```python
from build123d import *

# Parameters (mm, degrees)
BOSS_EXTRUDE1_DEPTH = 400
BOSS_EXTRUDE2_DEPTH = 10
SKETCH3_R           = 43.000999871
CUT_EXTRUDE1_DEPTH  = 447.360216168
BOSS_EXTRUDE3_DEPTH = 7
SKETCH5_R           = 1.75
CUT_EXTRUDE2_DEPTH  = 33
SKETCH6_W           = 36.000000185
SKETCH6_H           = 60
BOSS_EXTRUDE4_DEPTH = 5
SKETCH7_W           = 7.24997928
SKETCH7_H           = 16
BOSS_EXTRUDE5_DEPTH = 53
SKETCH8_W           = 12.24997928
SKETCH8_H           = 60
BOSS_EXTRUDE6_DEPTH = 5
FILLET1_R           = 5
SKETCH10_W          = 20.000000185
SKETCH10_H          = 40
BOSS_EXTRUDE7_DEPTH = 7.24997928
CUT_EXTRUDE3_DEPTH  = 6
CUT_EXTRUDE4_DEPTH  = 68.845857758
SKETCH12_R          = 4.5
CUT_EXTRUDE5_DEPTH  = 16
CHAMFER2_SIZE       = 5
CHAMFER3_SIZE       = 5
SKETCH13_R          = 6.5
SKETCH13_R_2        = 4.5
BOSS_EXTRUDE8_DEPTH = 2
FILLET2_R           = 1


with BuildPart() as part:
    # Sketch1 → Boss-Extrude1 (new body)
    with BuildSketch(Plane(origin=(0, 200, 0), x_dir=(1, 0, 0), z_dir=(0, 1, 0))):
        with BuildLine():
            Line((1e-09, -3.855700002), (0.25, -4.00003757))
            Line((0.25, -4.00003757), (9.078700232, -4.00003757))
            ThreePointArc((9.078700232, -4.00003757), (9.652725366, -4.114218268), (10.139360377, -4.439377387))
            Line((10.139360377, -4.439377387), (12.500020747, -6.800037757))
            Line((12.500020747, -6.800037757), (12.500020747, -9.500037757))
            Line((12.500020747, -9.500037757), (13.00002072, -10.000037755))
            Line((13.00002072, -10.000037755), (17.00002072, -10.000037755))
            Line((17.00002072, -10.000037755), (17.500020747, -9.500037752))
            Line((17.500020747, -9.500037752), (17.500020747, -5.500037752))
            Line((17.500020747, -5.500037752), (17.00002075, -5.0000377))
            Line((17.00002075, -5.0000377), (14.30002072, -5.0000377))
            Line((14.30002072, -5.0000377), (14.085807141, -4.785824121))
            ThreePointArc((14.085807141, -4.785824121), (13.652261651, -4.136977442), (13.50002072, -3.371610598))
            Line((13.50002072, -3.371610598), (13.50002072, -0.30003757))
            Line((13.50002072, -0.30003757), (13.20002072, -3.757e-05))
            Line((13.20002072, -3.757e-05), (7.50002072, -3.757e-05))
            Line((7.50002072, -3.757e-05), (7.40002072, -0.10003757))
            Line((7.40002072, -0.10003757), (-7.40002072, -0.10003757))
            Line((-7.40002072, -0.10003757), (-7.50002072, -3.757e-05))
            Line((-7.50002072, -3.757e-05), (-13.20002072, -3.757e-05))
            Line((-13.20002072, -3.757e-05), (-13.50002072, -0.30003757))
            Line((-13.50002072, -0.30003757), (-13.50002072, -3.371610628))
            ThreePointArc((-13.50002072, -3.371610628), (-13.652261651, -4.136977472), (-14.085807141, -4.785824151))
            Line((-14.085807141, -4.785824151), (-14.30002069, -5.0000377))
            Line((-14.30002069, -5.0000377), (-17.00002072, -5.0000377))
            Line((-17.00002072, -5.0000377), (-17.50002072, -5.50003767))
            Line((-17.50002072, -5.50003767), (-17.50002072, -9.50003767))
            Line((-17.50002072, -9.50003767), (-17.000020665, -10.000037755))
            Line((-17.000020665, -10.000037755), (-13.00002072, -10.000037755))
            Line((-13.00002072, -10.000037755), (-12.500020741, -9.500037764))
            Line((-12.500020741, -9.500037764), (-12.500020741, -6.800037764))
            Line((-12.500020741, -6.800037764), (-10.139360364, -4.439377387))
            ThreePointArc((-10.139360364, -4.439377387), (-9.652725352, -4.114218268), (-9.078700218, -4.00003757))
            Line((-9.078700218, -4.00003757), (-0.25, -4.00003757))
            Line((-0.25, -4.00003757), (1e-09, -3.855700002))
        make_face()
    extrude(amount=-BOSS_EXTRUDE1_DEPTH)

    # Sketch3 → Cut-Extrude1 (cut)
    with BuildSketch(Plane(origin=(0, 200, 0), x_dir=(1, 0, 0), z_dir=(0, 1, 0))):
        with Locations((0, -0.10003757)):
            Circle(SKETCH3_R)
    extrude(amount=-CUT_EXTRUDE1_DEPTH, mode=Mode.SUBTRACT)


with BuildPart() as body_2:
    # Sketch2 → Boss-Extrude2 (new body)
    with BuildSketch(Plane(origin=(0, 210, 0), x_dir=(1, 0, 0), z_dir=(0, 1, 0))):
        Polygon((-8.353826469, -7.25003757), (8.353826482, -7.25003757), (9.250020747, -8.146231835), (9.250020747, -10.846231788), (11.653826595, -13.250037755), (18.34621475, -13.250037755), (20.750020747, -10.846231878), (20.750020747, -4.153843779), (18.346214932, -1.7500377), (16.75002072, -1.7500377), (16.75002072, 1.046156508), (14.546214798, 3.24996243), (-14.546214798, 3.24996243), (-16.75002072, 1.046156508), (-16.75002072, -1.7500377), (-18.346214741, -1.7500377), (-20.75002072, -4.153843535), (-20.75002072, -10.846231691), (-18.3462148, -13.250037755), (-11.653826621, -13.250037755), (-9.250020741, -10.846231821), (-9.250020741, -8.146231842), align=None)
        with BuildLine():
            Line((13.303574111, 0.24996243), (-13.303574111, 0.24996243))
            Line((-13.303574111, 0.24996243), (-13.75002072, -0.196484179))
            Line((-13.75002072, -0.196484179), (-13.75002072, -3.371610628))
            ThreePointArc((-13.75002072, -3.371610628), (-13.883231534, -4.041306614), (-14.262583837, -4.609047456))
            Line((-14.262583837, -4.609047456), (-14.403574081, -4.7500377))
            Line((-14.403574081, -4.7500377), (-17.103574106, -4.7500377))
            Line((-17.103574106, -4.7500377), (-17.75002072, -5.396484275))
            Line((-17.75002072, -5.396484275), (-17.75002072, -9.603591056))
            Line((-17.75002072, -9.603591056), (-17.10357406, -10.250037755))
            Line((-17.10357406, -10.250037755), (-12.896467328, -10.250037755))
            Line((-12.896467328, -10.250037755), (-12.250020741, -9.603591153))
            Line((-12.250020741, -9.603591153), (-12.250020741, -6.903591155))
            Line((-12.250020741, -6.903591155), (-9.962583668, -4.616154083))
            ThreePointArc((-9.962583668, -4.616154083), (-9.557054494, -4.345188152), (-9.078700218, -4.25003757))
            Line((-9.078700218, -4.25003757), (9.078700232, -4.25003757))
            ThreePointArc((9.078700232, -4.25003757), (9.557054508, -4.345188152), (9.962583682, -4.616154083))
            Line((9.962583682, -4.616154083), (12.250020747, -6.903591148))
            Line((12.250020747, -6.903591148), (12.250020747, -9.603591144))
            Line((12.250020747, -9.603591144), (12.896467326, -10.250037755))
            Line((12.896467326, -10.250037755), (17.103574107, -10.250037755))
            Line((17.103574107, -10.250037755), (17.750020747, -9.603591147))
            Line((17.750020747, -9.603591147), (17.750020747, -5.39648437))
            Line((17.750020747, -5.39648437), (17.103574149, -4.7500377))
            Line((17.103574149, -4.7500377), (14.403574111, -4.7500377))
            Line((14.403574111, -4.7500377), (14.262583837, -4.609047426))
            ThreePointArc((14.262583837, -4.609047426), (13.883231534, -4.041306584), (13.75002072, -3.371610598))
            Line((13.75002072, -3.371610598), (13.75002072, -0.196484179))
            Line((13.75002072, -0.196484179), (13.303574111, 0.24996243))
        make_face(mode=Mode.SUBTRACT)
    extrude(amount=BOSS_EXTRUDE2_DEPTH)

    # Sketch4 → Boss-Extrude3 (add)
    with BuildSketch(Plane(origin=(0, 210, 0), x_dir=(-1, 0, 0), z_dir=(0, -1, 0))):
        Polygon((27, -13.250037755), (27, 22.74996243), (-27, 22.74996243), (-27, -13.250037755), (-18.34621475, -13.250037755), (-20.750020747, -10.846231878), (-20.750020747, -4.153843779), (-18.346214932, -1.7500377), (-16.75002072, -1.7500377), (-16.75002072, 1.046156508), (-14.546214798, 3.24996243), (14.546214798, 3.24996243), (16.75002072, 1.046156508), (16.75002072, -1.7500377), (18.346214741, -1.7500377), (20.75002072, -4.153843535), (20.75002072, -10.846231691), (18.3462148, -13.250037755), align=None)
    extrude(amount=-BOSS_EXTRUDE3_DEPTH)

    # Sketch5 → Cut-Extrude2 (cut)
    with BuildSketch(Plane(origin=(0, 210, 0), x_dir=(-1, 0, 0), z_dir=(0, -1, 0))):
        with Locations(Location((22.5, 18.24996243, 0), (0, 0, 90))):
            Circle(SKETCH5_R)
        with Locations(Location((22.5, 8.24996243, 0), (0, 0, 90))):
            Circle(SKETCH5_R)
        with Locations(Location((-22.5, 8.24996243, 0), (0, 0, 90))):
            Circle(SKETCH5_R)
        with Locations(Location((-22.5, 18.24996243, 0), (0, 0, 90))):
            Circle(SKETCH5_R)
    extrude(amount=-CUT_EXTRUDE2_DEPTH, mode=Mode.SUBTRACT)

    # Sketch6 → Boss-Extrude4 (add)
    with BuildSketch(Plane.ZY.offset(27)):
        with Locations((-4.749962337, 240)):
            Rectangle(SKETCH6_W, SKETCH6_H)
    extrude(amount=BOSS_EXTRUDE4_DEPTH)

    # Sketch7 → Boss-Extrude5 (add)
    with BuildSketch(Plane(origin=(0, 217, 0), x_dir=(1, 0, 0), z_dir=(0, 1, 0))):
        with Locations((-23.37501036, -5.250037755)):
            Rectangle(SKETCH7_W, SKETCH7_H)
    extrude(amount=BOSS_EXTRUDE5_DEPTH)

    # Sketch8 → Boss-Extrude6 (add)
    with BuildSketch(Plane(origin=(0, 0, -22.74996243), x_dir=(-1, 0, 0), z_dir=(0, 0, -1))):
        with Locations((25.87501036, 240)):
            Rectangle(SKETCH8_W, SKETCH8_H)
    extrude(amount=BOSS_EXTRUDE6_DEPTH)

    # Fillet1
    fillet1_edges = [body_2.edges().sort_by_distance(p)[0] for p in [
        (-19.75002072, 213.5, -22.74996243),
    ]]
    fillet(fillet1_edges, radius=FILLET1_R - 0.0001)  # a hair under: the kernel refuses the full size

    # Sketch10 → Boss-Extrude7 (add)
    with BuildSketch(Plane(origin=(-27, 0, 0), x_dir=(0, 0, -1), z_dir=(1, 0, 0))):
        with Locations((12.749962337, 250)):
            Rectangle(SKETCH10_W, SKETCH10_H)
    extrude(amount=BOSS_EXTRUDE7_DEPTH)

    # Sketch9 → Cut-Extrude3 (cut)
    with BuildSketch(Plane(origin=(-19.75002072, 0, 0), x_dir=(0, 0, -1), z_dir=(1, 0, 0))):
        Polygon((14.755515837, 250), (11.002739087, 256.5), (3.497185588, 256.5), (-0.255591162, 250), (3.497185588, 243.5), (11.002739087, 243.5), align=None)
    extrude(amount=-CUT_EXTRUDE3_DEPTH, mode=Mode.SUBTRACT)

    # Sketch11 → Cut-Extrude4 (cut, through all)
    with BuildSketch(Plane(origin=(0, 217, 0), x_dir=(1, 0, 0), z_dir=(0, 1, 0))):
        with BuildLine():
            Line((-22.5, 20.74996243), (-17.824832595, 20.74996243))
            Line((-17.824832595, 20.74996243), (-17.824832595, 15.74996243))
            Line((-17.824832595, 15.74996243), (-22.5, 15.74996243))
            ThreePointArc((-22.5, 15.74996243), (-25, 18.24996243), (-22.5, 20.74996243))
        make_face()
        with BuildLine():
            Line((-22.5, 10.74996243), (-17.824832595, 10.74996243))
            Line((-17.824832595, 10.74996243), (-17.824832595, 5.74996243))
            Line((-17.824832595, 5.74996243), (-22.5, 5.74996243))
            ThreePointArc((-22.5, 5.74996243), (-25, 8.24996243), (-22.5, 10.74996243))
        make_face()
    extrude(amount=CUT_EXTRUDE4_DEPTH, mode=Mode.SUBTRACT)

    # Sketch12 → Cut-Extrude5 (cut)
    with BuildSketch(Plane(origin=(-25.75002072, 0, 0), x_dir=(0, 0, -1), z_dir=(1, 0, 0))):
        with Locations((7.249962338, 250)):
            Circle(SKETCH12_R)
    extrude(amount=-CUT_EXTRUDE5_DEPTH, mode=Mode.SUBTRACT)

    # Chamfer2
    chamfer2_edges = [body_2.edges().sort_by_distance(p)[0] for p in [
        (-32, 270, -7.249962337),
    ]]
    chamfer(chamfer2_edges, length=CHAMFER2_SIZE)

    # Chamfer3
    chamfer3_edges = [body_2.edges().sort_by_distance(p)[0] for p in [
        (-32, 210, -7.249962338),
    ]]
    chamfer(chamfer3_edges, length=CHAMFER3_SIZE)

    # Sketch13 → Boss-Extrude8 (add)
    with BuildSketch(Plane.ZY.offset(32)):
        with Locations(Location((-7.249962338, 250, 0), (0, 0, 180))):
            Circle(SKETCH13_R)
        with Locations(Location((-7.249962338, 250, 0), (0, 0, 180))):
            Circle(SKETCH13_R_2, mode=Mode.SUBTRACT)
    extrude(amount=BOSS_EXTRUDE8_DEPTH)

    # Fillet2
    fillet2_edges = [body_2.edges().sort_by_distance(p)[0] for p in [
        (-32, 250, -0.749962338),
    ]]
    fillet(fillet2_edges, radius=FILLET2_R)


solid = body_2.part
```
CAD build for the part. Positions are in the model's coordinates, mm. A direction names the side the tool comes from. Give positions to 0.01 mm unless a question says otherwise; leave off trailing zeros. Order: outer loops, then holes, each group sorted by start corner. A loop starts at its lowest first (then second) coordinate and runs counter-clockwise, first axis right, second up. Notation, with made-up numbers: M 10.25,57 L 22.25,57 A11 cw 22.25,73 Z; hole C 0.5,-15.5 d4. An arc over 180 degrees is marked long. Put each result on its own line as item: value. Start each with the question number.
(1) Saw through at B-B, the plane y = 266. Write the cut outline in (x, z).
(2) Saw through at A-A, the plane x = -2. Write the cut outline in (y, z), then the cut area to 4 significant figures.
(3) Saw through at D-D, the plane z = -8. Give the number of separate pieces and of enclosed holes in the cut face, then the cut area to 3 significant figures.
(4) Mould opens along Z. For faces 4 (the cylindrical face through (-25, 249.7, -18.2)), 5 (the flat face through (9.25, 215, 9)), 6 (the flat face through (0, 215, 7.25)) say: +Z half, -Z half, draft (parallel to the pull), parting line (faces both ways), or undercut.
(5) Which spindle directions (+Z, -Z, +X, -X, +Y, -Y) get a long thin tool onto all of the face, cutting with end or side? Do faces 1 (the flat face through (18, 218, 1.75)), 2 (the flat face through (-22.71, 246.8, -1.59)), 3 (the cylindrical face through (-25, 236.7, -8.2)). Say none if no direction does.
(6) Saw through at C-C, the plane x = 22.5. Write the cut outline in (y, z), then the cut area to 3 significant figures.
(7) Flat gauge pins, fed straight in: pin 1 Ø5.5 at (y, z) = (239, 3.5) entering from +X; pin 2 Ø10 at (x, y) = (14, 226.5) entering from -Z; pin 3 Ø4 at (y, z) = (220, -7) entering from +X; pin 4 Ø0.8 at (x, y) = (18, 218) entering from -Z. Where does each tip first touch, or does it go through?
(8) Drill centre lines: line 1 along Z through (x, y) = (-22, 215); line 2 along Z through (x, y) = (-20.5, 224.5); line 3 along Y through (x, z) = (15.5, 2). Where is each one in solid material? Low to high.
Check result:
1. outline: M -31,-27.75 L -19.75,-27.75 L -19.75,-20.75 L -22.5,-20.75 A2.5 cw -22.5,-15.75 L -19.75,-15.75 L -19.75,-10.75 L -22.5,-10.75 A2.5 cw -22.5,-5.75 L -19.75,-5.75 L -19.75,13.25 L -31,13.25 Z
2. outline: M 210,-22.75 L 217,-22.75 L 217,-3.25 L 220,-3.25 L 220,-0.25 L 210,-0.25 Z; M 210,4.25 L 220,4.25 L 220,7.25 L 210,7.25 Z
2. area: 196.5 mm2
3. separate pieces: 4
3. enclosed holes: 0
3. area: 628 mm2
4. face 4: undercut
4. face 5: draft
4. face 6: +Z half
5. face 1: -Z, +X, +Y
5. face 2: +X
5. face 3: +X, +Y
6. outline: M 210,-22.75 L 217,-22.75 L 217,-20 L 210,-20 Z; M 210,-16.5 L 217,-16.5 L 217,-10 L 210,-10 Z; M 210,-6.5 L 217,-6.5 L 217,13.25 L 210,13.25 Z
6. area: 203 mm2
7. pin 1: stops at x = -19.75
7. pin 2: passes through
7. pin 3: stops at x = -27
7. pin 4: stops at z = 1.75
8. line 1: z = -27.75 to -19.93, -16.57 to -9.93, -6.57 to 13.25
8. line 2: z = -27.75 to -22.75, -2.75 to 13.25
8. line 3: y = 210 to 220
